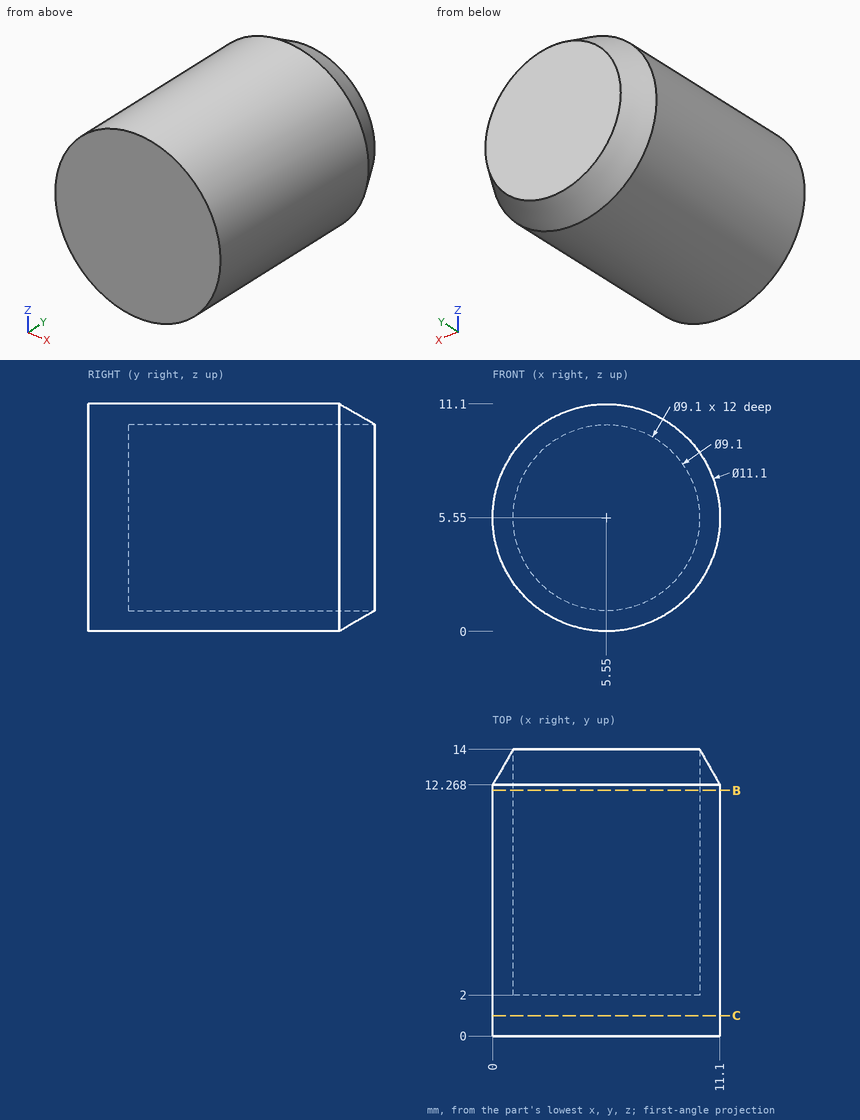
Check sheet for the drawn part. Datum: minimum x, y, z corner. Units: mm. Round coordinates to 2 decimals unless told otherwise and drop trailing zeros. Order: outer loops, then holes, each group sorted by start corner. A loop starts at its lowest first (then second) coordinate and runs counter-clockwise, first axis right, second up. Notation, with made-up numbers: (11.25, 88.25) - (24.25, 88.25) arc R24 cw to (24.25, 114.25) - close; hole circle Ø4 at (28.25, 4). An arc over 180 degrees is marked (long way). Use a Markdown table: item, result. Add a question column.
(1) Material ranges on line 1 along Z through (x, y) = (5.55, 10); line 2 along Y through (x, z) = (3.5, 8.75); line 3 along X through (y, z) = (2.5, 8.25), recorded low to high. Write a range as [from, to].
(2) Sectioned sample at C-C, the plane y = 1. Enter the section's corners in (x, z).
(3) Depth check by flat-ended pin: pin 1 (5 mm diameter, centred on y = 12.5, z = 8.5, fed in from +X); pin 2 (1.5 mm diameter, centred on x = 3, y = 6, fed in from +Z); pin 3 (4 mm diameter, centred on x = 1.5, y = 11.5, fed in from -Z). Enter the tip coordinate at first touch or a pass-through.
(4) Sectioned sample at B-B, the plane y = 12. Enter the section's corners in (x, z).
Answers below:
| question | item | result |
|---|---|---|
| 1 | line 1 | [0, 1], [10.1, 11.1] |
| 1 | line 2 | [0, 2] |
| 1 | line 3 | [0.7, 1.89], [9.21, 10.4] |
| 2 | outline | circle Ø11.1 at (5.55, 5.55) |
| 3 | pin 1 | x = 11.08 |
| 3 | pin 2 | z = 10.8 |
| 3 | pin 3 | z = 0.39 |
| 4 | outline | circle Ø11.1 at (5.55, 5.55); hole circle Ø9.1 at (5.55, 5.55) |
